Verification items for the finished model (mm, model axes). Face numbers are marked on the shaded views. Coordinates: 2 decimals unless noted, no trailing zeros. Loops run counter-clockwise (first coordinate to the right, second up) from the corner with the lowest first, then second, coordinate; pieces in that order, holes last.
Q1. Sectioned sample at D-D (y = -69). Enter the section's corners in (x, z).
Q2. Material ranges on probe 1 along Z at (x, y) = (0, -25); probe 2 along Z at (x, y) = (21, -50); probe 3 along X at (y, z) = (-39, -4), recorded low to high.
Q3. Mould release check, pull along Z, two halves, no side actions. Record for the marked faces 1, 2 and 3: +Z half, -Z half, draft (parallel to the pull), parting line (faces both ways), or undercut.
Q4. Sectioned sample at C-C (x = 0). Enter the section's corners in (y, z), then the cut area to 3 significant figures.
Q5. Sectioned sample at A-A (z = 0). Enter the section's corners in (x, y), then the cut area to 3 significant figures.
Q6. Sectioned sample at B-B (y = -53). Enter the section's corners in (x, z).
Q7. Go/stop test with a flat-tipped pin: P1, Ø5, axis at x = -12.5, z = 30, coming from the -Y side. Record where the tip stops, or that it passes through.
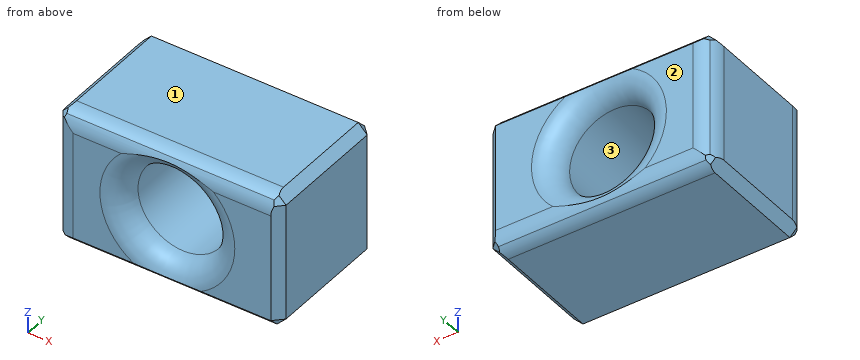
```python
from build123d import *

# Parameters (mm, degrees)
F0_W        = 127
F0_H        = 76.2
F0_R        = 25.4
F1_DEPTH    = 76.2
F2_SIZE     = 5.08
F3_T1_DEPTH = 143.1425612107
F3_T3_DEPTH = 92.3425612107


# Not quite as in the source:
# - a fillet or chamfer that OpenCascade refuses, or shapes differently, is made with other operations: its cross-section is extruded or revolved along the edge and cut away or added


with BuildPart() as f1:
    # F0 (on Front) → F1 (new body)
    with BuildSketch(Plane.XZ):
        Rectangle(F0_W, F0_H)
        Circle(F0_R, mode=Mode.SUBTRACT)
    extrude(amount=F1_DEPTH)

    # F2
    f2_edges = [f1.edges().sort_by_distance(p)[0] for p in [
        (0, -76.2, 38.1),
        (-63.5, -38.1, 38.1),
        (0, 0, 38.1),
        (63.5, -38.1, 38.1),
        (63.5, -76.2, 0),
        (0, -76.2, -38.1),
        (-63.5, -76.2, 0),
        (63.5, -38.1, -38.1),
        (63.5, 0, 0),
        (0, 0, -38.1),
        (-63.5, 0, 0),
        (-63.5, -38.1, -38.1),
    ]]
    chamfer(f2_edges, length=F2_SIZE)

    # F3: fillet of radius 12.7 on 10 edges, made by hand

    # F3_s2 → F3_t1 (cut)
    with BuildSketch(Plane.YZ.offset(-71.5712806053)):
        with BuildLine():
            ThreePointArc((0, -27.7594877579), (-0.9667299371, -32.6195673489), (-3.7197438789, -36.7397438789))
            Line((-3.7197438789, -36.7397438789), (0, -33.02))
            Line((0, -33.02), (0, -27.7594877579))
        make_face()
        with BuildLine():
            ThreePointArc((-1.3602561211, -34.3802561211), (-5.4804326511, -37.1332700629), (-10.3405122421, -38.1))
            Line((-10.3405122421, -38.1), (-5.08, -38.1))
            Line((-5.08, -38.1), (-1.3602561211, -34.3802561211))
        make_face()
        with BuildLine():
            ThreePointArc((-65.8594877579, 38.1), (-70.7195673489, 37.1332700629), (-74.8397438789, 34.3802561211))
            Line((-74.8397438789, 34.3802561211), (-71.12, 38.1))
            Line((-71.12, 38.1), (-65.8594877579, 38.1))
        make_face()
        with BuildLine():
            ThreePointArc((-72.4802561211, 36.7397438789), (-75.2332700629, 32.6195673489), (-76.2, 27.7594877579))
            Line((-76.2, 27.7594877579), (-76.2, 33.02))
            Line((-76.2, 33.02), (-72.4802561211, 36.7397438789))
        make_face()
    extrude(amount=F3_T1_DEPTH, mode=Mode.SUBTRACT)

    # F3_s4 → F3_t3 (cut)
    with BuildSketch(Plane.XY.offset(-46.1712806053)):
        with BuildLine():
            ThreePointArc((-63.5, -65.8594877579), (-62.5332700629, -70.7195673489), (-59.7802561211, -74.8397438789))
            Line((-59.7802561211, -74.8397438789), (-63.5, -71.12))
            Line((-63.5, -71.12), (-63.5, -65.8594877579))
        make_face()
        with BuildLine():
            ThreePointArc((-53.1594877579, -76.2), (-58.0195673489, -75.2332700629), (-62.1397438789, -72.4802561211))
            Line((-62.1397438789, -72.4802561211), (-58.42, -76.2))
            Line((-58.42, -76.2), (-53.1594877579, -76.2))
        make_face()
        with BuildLine():
            ThreePointArc((-63.5, -10.3405122421), (-62.5332700629, -5.4804326511), (-59.7802561211, -1.3602561211))
            Line((-59.7802561211, -1.3602561211), (-63.5, -5.08))
            Line((-63.5, -5.08), (-63.5, -10.3405122421))
        make_face()
        with BuildLine():
            ThreePointArc((-53.1594877579, 0), (-58.0195673489, -0.9667299371), (-62.1397438789, -3.7197438789))
            Line((-62.1397438789, -3.7197438789), (-58.42, 0))
            Line((-58.42, 0), (-53.1594877579, 0))
        make_face()
    extrude(amount=F3_T3_DEPTH, mode=Mode.SUBTRACT)

    # F3_s5 → F3_t6 (revolve, cut)
    with BuildSketch(Plane.XY):
        with BuildLine():
            ThreePointArc((38.1, -76.2), (29.1197438789, -72.4802561211), (25.4, -63.5))
            Line((25.4, -63.5), (25.4, -76.2))
            Line((25.4, -76.2), (38.1, -76.2))
        make_face()
    revolve(axis=Axis((0, -76.2, 0), (0, -1, 0)), mode=Mode.SUBTRACT)

    # F3_s7 → F3_t8 (revolve, cut)
    with BuildSketch(Plane.XY):
        with BuildLine():
            ThreePointArc((38.1, 0), (29.1197438789, -3.7197438789), (25.4, -12.7))
            Line((25.4, -12.7), (25.4, 0))
            Line((25.4, 0), (38.1, 0))
        make_face()
    revolve(axis=Axis((0, 0, 0), (0, -1, 0)), mode=Mode.SUBTRACT)


solid = f1.part
```
Geometry check:
1. outline: (-63.11, -33.41) - (-58.42, -38.1) - (58.42, -38.1) - (63.5, -33.02) - (63.5, 33.02) - (58.81, 37.71) - (-58.81, 37.71) - (-63.11, 33.41) - close; hole circle Ø53.31 at (0, 0)
2. probe 1: z = -38.1 to -25.4, 25.4 to 38.1
2. probe 2: z = -38.1 to -14.29, 14.29 to 38.1
2. probe 3: x = -63.5 to -25.08, 25.08 to 63.5
3. face 1: +Z half
3. face 2: draft
3. face 3: undercut
4. outline: (-75.44, -33.78) - (-71.12, -38.1) - (-10.34, -38.1) arc R12.7 ccw to (-2.62, -35.48) arc R12.7 ccw to (-1.1, -32.93) arc R12.7 ccw to (-12.7, -25.4) - (-63.5, -25.4) arc R12.7 ccw to start; (-75.1, 32.93) arc R12.7 ccw to (-63.5, 25.4) - (-12.7, 25.4) arc R12.7 ccw to (-0.76, 33.78) - (-5.08, 38.1) - (-65.86, 38.1) arc R12.7 ccw to (-73.58, 35.48) arc R12.7 ccw to start
4. area: 1,740 mm2
5. outline: (-63.5, -65.86) arc R12.7 ccw to (-60.88, -73.58) arc R12.7 ccw to (-53.16, -76.2) - (-38.1, -76.2) arc R12.7 ccw to (-25.4, -63.5) - (-25.4, -12.7) arc R12.7 ccw to (-38.1, 0) - (-53.16, 0) arc R12.7 ccw to (-60.88, -2.62) arc R12.7 ccw to (-63.5, -10.34) - close; (25.4, -63.5) arc R12.7 ccw to (38.1, -76.2) - (58.42, -76.2) - (63.5, -71.12) - (63.5, -5.08) - (58.42, 0) - (38.1, 0) arc R12.7 ccw to (25.4, -12.7) - close
5. area: 5,600 mm2
6. outline: (-63.5, -33.02) - (-58.42, -38.1) - (58.42, -38.1) - (63.5, -33.02) - (63.5, 33.02) - (58.42, 38.1) - (-58.42, 38.1) - (-63.5, 33.02) - close; hole circle Ø50.8 at (0, 0)
7. P1: stops at y = -75.7
